```python
from build123d import *

# Parameters (mm, degrees)
SKETCH1_W             = 177.8
SKETCH1_H             = 157.988
BASE_FLANGE1_DEPTH    = 2.54
CUT_EXTRUDE1_DEPTH    = 238.864456664
F_4_40_TAPPED_HOLE1_D = 2.2606
LPATTERN1_COUNT       = 5
LPATTERN1_PITCH       = 31.75
EDGE_FLANGE1_DEPTH    = 177.8
EDGE_FLANGE2_DEPTH    = 177.8
CUT_EXTRUDE4_REACH    = 256.794
LPATTERN2_COUNT       = 4
LPATTERN2_PITCH       = 31.75
CUT_EXTRUDE5_REACH    = 263.778
SKETCH28_W            = 6.604
SKETCH28_H            = 6.604
CUT_EXTRUDE3_REACH    = 256.794
SKETCH24_R            = 6.35


# Sheet-metal steps are written as plain solids
with BuildPart() as part:
    # Sketch1 → Base-Flange1 (new body)
    with BuildSketch(Plane.XY):
        with Locations((88.9, 78.994)):
            Rectangle(SKETCH1_W, SKETCH1_H)
    extrude(amount=-BASE_FLANGE1_DEPTH)

    # Sketch6 → Cut-Extrude1 (cut, through all)
    with BuildSketch(Plane.XY):
        with BuildLine():
            Line((20.0025, 17.89176), (30.7975, 17.89176))
            ThreePointArc((30.7975, 17.89176), (32.593551224, 18.635708776), (33.3375, 20.43176))
            Line((33.3375, 20.43176), (33.3375, 66.15176))
            ThreePointArc((33.3375, 66.15176), (32.593551224, 67.947811224), (30.7975, 68.69176))
            Line((30.7975, 68.69176), (20.0025, 68.69176))
            ThreePointArc((20.0025, 68.69176), (18.206448776, 67.947811224), (17.4625, 66.15176))
            Line((17.4625, 66.15176), (17.4625, 20.43176))
            ThreePointArc((17.4625, 20.43176), (18.206448776, 18.635708776), (20.0025, 17.89176))
        make_face()
    cut_extrude1 = extrude(amount=-CUT_EXTRUDE1_DEPTH, mode=Mode.SUBTRACT)

    # #4-40 Tapped Hole1 (through all)
    with Locations(Plane(origin=(23.8125, 141.824456, 0), x_dir=(1, 0, 0), z_dir=(0, 0, 1))):
        with Locations((0, 0), (0, -19.05)):
            f_4_40_tapped_hole1 = Hole(F_4_40_TAPPED_HOLE1_D / 2)

    # LPattern1: Cut-Extrude1, #4-40 Tapped Hole1 ×5
    with Locations(*[(i * LPATTERN1_PITCH, 0, 0) for i in range(1, LPATTERN1_COUNT)]):
        add(cut_extrude1, mode=Mode.SUBTRACT)
        add(f_4_40_tapped_hole1, mode=Mode.SUBTRACT)

    # Edge-Flange1 section (across the edge) → Edge-Flange1 (add)
    with BuildSketch(Plane(origin=(0, 160.187704526, -2.54), x_dir=(0, -0.8660254037844364, -0.5000000000000041), z_dir=(1, 0, 0))):
        with BuildLine():
            Line((-2.54, 2.199704526), (-2.54, 26.473530316))
            Line((-2.54, 26.473530316), (0, 26.473530316))
            Line((0, 26.473530316), (0, 2.199704526))
            ThreePointArc((0, 2.199704526), (0.510443212, 0.294704526), (1.905, -1.099852263))
            Line((1.905, -1.099852263), (0.635, -3.299556788))
            ThreePointArc((0.635, -3.299556788), (-1.689261314, -0.975295474), (-2.54, 2.199704526))
        make_face()
    extrude(amount=EDGE_FLANGE1_DEPTH)

    # Edge-Flange2 section (across the edge) → Edge-Flange2 (add)
    with BuildSketch(Plane(origin=(177.8, -6.599113577, -2.54), x_dir=(0, 0.8660254037844398, 0.499999999999998), z_dir=(-1, 0, 0))):
        with BuildLine():
            Line((-2.54, 6.599113577), (-2.54, 65.450590949))
            Line((-2.54, 65.450590949), (0, 65.450590949))
            Line((0, 65.450590949), (0, 6.599113577))
            ThreePointArc((0, 6.599113577), (1.905, 3.299556788), (5.715, 3.299556788))
            Line((5.715, 3.299556788), (6.985, 1.099852263))
            ThreePointArc((6.985, 1.099852263), (0.635, 1.099852263), (-2.54, 6.599113577))
        make_face()
    extrude(amount=EDGE_FLANGE2_DEPTH)

    # Sketch25 → Cut-Extrude4 (cut, up to next)
    with BuildSketch(Plane(origin=(0, 121.240630657, 69.998310747), x_dir=(1, 0, 0), z_dir=(0, 0.8660254037844362, 0.5000000000000044)), mode=Mode.PRIVATE) as cut_extrude4_sk1:
        with BuildLine():
            Line((33.401, 97.337087105), (49.149, 97.337087105))
            ThreePointArc((49.149, 97.337087105), (49.86742049, 97.039507594), (50.165, 96.321087105))
            Line((50.165, 96.321087105), (50.165, 90.733087105))
            ThreePointArc((50.165, 90.733087105), (49.86742049, 90.014666615), (49.149, 89.717087105))
            Line((49.149, 89.717087105), (33.401, 89.717087105))
            ThreePointArc((33.401, 89.717087105), (32.68257951, 90.014666615), (32.385, 90.733087105))
            Line((32.385, 90.733087105), (32.385, 96.321087105))
            ThreePointArc((32.385, 96.321087105), (32.68257951, 97.039507594), (33.401, 97.337087105))
        make_face()
    cut_extrude4_tool1 = extrude(cut_extrude4_sk1.sketch, amount=-CUT_EXTRUDE4_REACH, mode=Mode.PRIVATE) & part.part
    cut_extrude4 = cut_extrude4_tool1.solids().sort_by_distance((41.275, 168.004174, -10.998523))[0]
    add(cut_extrude4, mode=Mode.SUBTRACT)

    # LPattern2: Cut-Extrude4 ×4
    with Locations(*[(i * LPATTERN2_PITCH, 0, 0) for i in range(1, LPATTERN2_COUNT)]):
        add(cut_extrude4, mode=Mode.SUBTRACT)

    # Sketch28 → Cut-Extrude5 (cut, up to next)
    with BuildSketch(Plane(origin=(0, -8.248891971, -4.7625), x_dir=(1, 0, 0), z_dir=(0, -0.8660254037844399, -0.49999999999999806)), mode=Mode.PRIVATE) as cut_extrude5_sk1:
        with Locations((25.4, -31.330738686)):
            Rectangle(SKETCH28_W, SKETCH28_H)
    cut_extrude5_tool1 = extrude(cut_extrude5_sk1.sketch, amount=-CUT_EXTRUDE5_REACH, mode=Mode.PRIVATE) & part.part
    # Sketch28 → Cut-Extrude5 (cut, up to next)
    with BuildSketch(Plane(origin=(0, -8.248891971, -4.7625), x_dir=(1, 0, 0), z_dir=(0, -0.8660254037844399, -0.49999999999999806)), mode=Mode.PRIVATE) as cut_extrude5_sk2:
        with Locations((152.4, -31.330738686)):
            Rectangle(SKETCH28_W, SKETCH28_H)
    cut_extrude5_tool2 = extrude(cut_extrude5_sk2.sketch, amount=-CUT_EXTRUDE5_REACH, mode=Mode.PRIVATE) & part.part
    add(cut_extrude5_tool1.solids().sort_by_distance((25.4, 7.416477, -31.895716))[0], mode=Mode.SUBTRACT)
    add(cut_extrude5_tool2.solids().sort_by_distance((152.4, 7.416477, -31.895716))[0], mode=Mode.SUBTRACT)

    # Sketch24 → Cut-Extrude3 (cut, up to next)
    with BuildSketch(Plane(origin=(0, 121.240630657, 69.998310747), x_dir=(1, 0, 0), z_dir=(0, 0.8660254037844362, 0.5000000000000044)), mode=Mode.PRIVATE) as cut_extrude3_sk1:
        with Locations(Location((13.335, 94.543087105, 0), (0, 0, 270))):
            Circle(SKETCH24_R)
    cut_extrude3_tool1 = extrude(cut_extrude3_sk1.sketch, amount=-CUT_EXTRUDE3_REACH, mode=Mode.PRIVATE) & part.part
    # Sketch24 → Cut-Extrude3 (cut, up to next)
    with BuildSketch(Plane(origin=(0, 121.240630657, 69.998310747), x_dir=(1, 0, 0), z_dir=(0, 0.8660254037844362, 0.5000000000000044)), mode=Mode.PRIVATE) as cut_extrude3_sk2:
        with Locations(Location((164.465, 94.543087105, 0), (0, 0, 270))):
            Circle(SKETCH24_R)
    cut_extrude3_tool2 = extrude(cut_extrude3_sk2.sketch, amount=-CUT_EXTRUDE3_REACH, mode=Mode.PRIVATE) & part.part
    add(cut_extrude3_tool1.solids().sort_by_distance((13.335, 168.512174, -11.878404))[0], mode=Mode.SUBTRACT)
    add(cut_extrude3_tool2.solids().sort_by_distance((164.465, 168.512174, -11.878404))[0], mode=Mode.SUBTRACT)


solid = part.part
```
For this review, take the finished solid that the model builds, in its own axes (mm). A direction names the side the tool comes from. Coordinates: 2 decimals unless noted, no trailing zeros. Write each loop counter-clockwise with the first axis right and the second up, starting at its lowest first coordinate (ties: lowest second). Pieces come first, ordered by that corner, then holes. Notation, with made-up numbers: (71.25, 21.25) - (111.25, 21.25) arc R26 cw to (111.25, 40.25) - close; hole circle Ø7 at (-18, 8.25). An arc over 180 degrees is marked (long way). Put each result on its own line as item: value.
1. Wall thickness on probe 1 along Y at (x, z) = (115, -9.5); probe 2 along Z at (x, y) = (32, 13.5); probe 3 along Y at (x, z) = (80, -16.5): over which ranges is each line inside the solid? List them lowest first.
Values found:
probe 1: -5.51 to -2.58, 164.21 to 167.14
probe 2: -42.43 to -37.35, -2.54 to 0
probe 3: -1.47 to 1.46, 168.25 to 171.18
2. Add section B-B, the plane y = 62.5. Give the boundary of the cut face in (x, z).
Values found:
outline: (0, -2.54) - (17.46, -2.54) - (17.46, 0) - (0, 0) - close; (33.34, -2.54) - (49.21, -2.54) - (49.21, 0) - (33.34, 0) - close; (65.09, -2.54) - (80.96, -2.54) - (80.96, 0) - (65.09, 0) - close; (96.84, -2.54) - (112.71, -2.54) - (112.71, 0) - (96.84, 0) - close; (128.59, -2.54) - (144.46, -2.54) - (144.46, 0) - (128.59, 0) - close; (160.34, -2.54) - (177.8, -2.54) - (177.8, 0) - (160.34, 0) - close
3. Add section D-D, the plane y = 115. Give the boundary of the cut face in (x, z).
Values found:
outline: (0, -2.54) - (177.8, -2.54) - (177.8, 0) - (0, 0) - close
4. Mouldability with a two-part tool opening along Z and no side actions: class faces 3 (the flat face through (50.165, 167, -12)), 4 (the cylindrical face through (90, -3, -4)), 5 (the cylindrical face through (87.655, 161.123, -0.828)), 6 (the flat face through (22.098, 9, -31)) as released by +Z, released by -Z, zero draft, split by the parting line, or undercut.
Values found:
face 3: zero draft
face 4: undercut
face 5: released by +Z
face 6: undercut
5. Add section A-A, the plane x = 131. Give the boundary of the cut face in (y, z) (3 decimals), then the cut area to 3 significant figures.
Values found:
outline: (-5.499, -9.525) - (23.926, -60.492) - (26.126, -59.222) - (-3.3, -8.255) arc R3.81 cw to (0, -2.54) - (157.988, -2.54) arc R3.81 cw to (161.288, -4.445) - (163.899, -8.969) - (166.099, -7.699) - (163.487, -3.175) arc R6.35 ccw to (157.988, 0) - (0, 0) arc R6.35 ccw to start; (167.709, -15.568) - (173.424, -25.467) - (175.624, -24.197) - (169.909, -14.298) - close
area: 634 mm²
6. Add section C-C, the plane z = -21. Give the boundary of the cut face in (x, y), then the cut area to 3 significant figures.
Values found:
outline: (0, 1.13) - (177.8, 1.13) - (177.8, 4.06) - (0, 4.06) - close; (0, 170.85) - (177.8, 170.85) - (177.8, 173.78) - (0, 173.78) - close
area: 1,040 mm²
7. For pin 1 (5 mm diameter, centred on x = 94, z = -40, fed in from -Y); pin 2 (1.3 mm diameter, centred on x = 123, z = -1, fed in from +Y); pin 3 (2 mm diameter, centred on x = 150.5, z = -0.5, fed in from +Y), all flat-tipped, find the tip position at first contact; note any pin that passes through.
Values found:
pin 1: y = 10.65
pin 2: y = 162.26
pin 3: y = 162.09
8. Machinability: for faces 1 (the flat face through (87.66, 169.47, -13.54)), 2 (the flat face through (90.14, 11.62, -34.1)), which of the approach directions +Z, -Z, +X, -X, +Y, -Y give a long, thin tool a straight path to every point of the face, cutting with its end or side? Answer none if there is none.
Values found:
face 1: +Z, +X, -X, +Y
face 2: +X, -X
